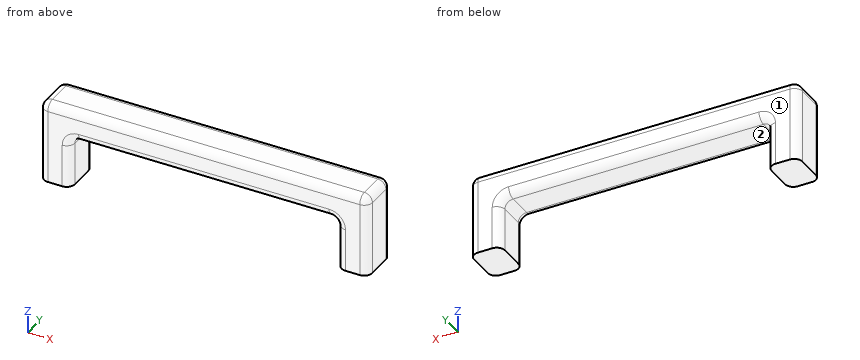
Autodesk Inventor part; units mm, degrees
ref_plane "YZ Plane" through (0, 0, 0) normal (1, 0, 0) x (0, 1, 0)
ref_plane "XZ Plane" through (0, 0, 0) normal (0, 1, 0) x (-1, 0, 0)
ref_plane "XY Plane" through (0, 0, 0) normal (0, 0, 1) x (1, 0, 0)
sketch "Sketch4" plane through (0, 0, 0) normal (0, 0, 1) x (1, 0, 0)
  line L0 (-80, 10) -> (80, 10)
  line L1 (80, 10) -> (80, -10)
  line L2 (80, -10) -> (-80, -10)
  line L3 (-80, -10) -> (-80, 10)
  line L4 (-80, 10) -> (80, -10) construction
  line L5 (80, 10) -> (-80, -10) construction
  point P0 (0, 0)
  dimension "d33" = 160
  dimension "d34" = 20
extrude "Extrusion1" add sketch "Sketch4" along normal blind 40
sketch "Sketch5" plane through (-80, 10, 0) normal (0, 1, 0) x (1, 0, 0)
  line L0 (0, 0) -> (160, 0)
  line L1 (15, 0) -> (145, 0)
  line L2 (145, 0) -> (145, -25)
  line L3 (145, -25) -> (15, -25)
  line L4 (15, -25) -> (15, 0)
  line L5 (160, -40) -> (0, -40)
  line L6 (160, 0) -> (160, -40)
  line L7 (0, 0) -> (0, -40)
  point P0 (80, 0)
  point P1 (0, -20)
  dimension "d37" = 15
  dimension "d38" = 15
  dimension "d39" = 15
extrude "Extrusion2" cut sketch "Sketch5" against normal blind 40 contours L0 L2 L3 L4
fillet "Fillet1" radius 4 16 edges at (80, 0, 40) (0, 10, 40) (0, -10, 40) (80, 10, 20) (80, -10, 20) (0, 10, 25) (65, 10, 12.5) (0, -10, 25) (65, -10, 12.5) (65, 0, 25) (-65, -10, 12.5) (-65, 0, 25) (-65, 10, 12.5) (-80, -10, 20) (-80, 10, 20) (-80, 0, 40)
properties part number "Handle"
Here's how the part is built. I have some questions about the finished solid (model axes, mm). Face numbers are marked on the shaded views. Coordinates: 2 decimals unless noted, no trailing zeros. Order: outer loops, then holes, each group sorted by start corner. A loop starts at its lowest first (then second) coordinate and runs counter-clockwise, first axis right, second up. Notation, with made-up numbers: (-19.5, -33.75) -> (25.5, -33.75) arc R7 cw to (25.5, -29.75) -> close; hole circle Ø9 at (25.25, -27.5). An arc over 180 degrees is marked (long way). Answer in a Markdown table with one row per item.
(1) Thinking about a two-plate mould opening in X: for the marked faces 1 and 2, which applies, +X half, -X half, draft (parallel to the pull), parting line (faces both ways), or undercut?
Answer key:
| item | result |
|---|---|
| face 1 | draft |
| face 2 | undercut |
(2) I want a section at A-A on z = 14.5. List the corners of the cut face in (x, y) for me.
Answer key:
| item | result |
|---|---|
| outline | (-80, -6) arc R4 ccw to (-76, -10) -> (-69, -10) arc R4 ccw to (-65, -6) -> (-65, 6) arc R4 ccw to (-69, 10) -> (-76, 10) arc R4 ccw to (-80, 6) -> close; (65, -6) arc R4 ccw to (69, -10) -> (76, -10) arc R4 ccw to (80, -6) -> (80, 6) arc R4 ccw to (76, 10) -> (69, 10) arc R4 ccw to (65, 6) -> close |
(3) I want a section at D-D on z = 37.5. List the corners of the cut face in (x, y) for me.
Answer key:
| item | result |
|---|---|
| outline | (-79.71, -6) arc R3.71 ccw to (-76, -9.71) -> (76, -9.71) arc R3.71 ccw to (79.71, -6) -> (79.71, 6) arc R3.71 ccw to (76, 9.71) -> (-76, 9.71) arc R3.71 ccw to (-79.71, 6) -> close |
(4) Please list where these lines run through material, in increasing order: probe 1 along X at (y, z) = (3.5, 8); probe 2 along Z at (x, y) = (-45, 6.5); probe 3 along X at (y, z) = (7.5, 8).
Answer key:
| item | result |
|---|---|
| probe 1 | -80 to -65, 65 to 80 |
| probe 2 | 25.03 to 39.97 |
| probe 3 | -79.71 to -65.29, 65.29 to 79.71 |
(5) Will this pin go through, and if not, where does the flat tip stop? pin 1 Ø9.5 at (x, y) = (4.5, -2.5) entering from -Z.
Answer key:
| item | result |
|---|---|
| pin 1 | z = 25 |
(6) I want a section at C-C on x = 7. List the corners of the cut face in (y, z) for me, then the cut area to 3 significant figures.
Answer key:
| item | result |
|---|---|
| outline | (-10, 29) arc R4 ccw to (-6, 25) -> (6, 25) arc R4 ccw to (10, 29) -> (10, 36) arc R4 ccw to (6, 40) -> (-6, 40) arc R4 ccw to (-10, 36) -> close |
| area | 286 mm^2 |
(7) I want a section at B-B on y = -4.25. List the corners of the cut face in (x, z) for me, then the cut area to 3 significant figures.
Answer key:
| item | result |
|---|---|
| outline | (-80, 0) -> (-65, 0) -> (-65, 21) arc R4 cw to (-61, 25) -> (61, 25) arc R4 cw to (65, 21) -> (65, 0) -> (80, 0) -> (80, 36) arc R4 ccw to (76, 40) -> (-76, 40) arc R4 ccw to (-80, 36) -> close |
| area | 3,150 mm^2 |
